```python
from build123d import *

# Parameters (mm, degrees)
F0_R     = 8
F1_DEPTH = 49
F3_D     = 4.2
F3_DEPTH = 17.4
F3_TIP   = 1.2618073
F5_D     = 4.2
F5_DEPTH = 17.4
F5_TIP   = 1.2618073


with BuildPart() as f1:
    # F0 (on Top) → F1 (new body)
    with BuildSketch(Plane.XY):
        Circle(F0_R)
    extrude(amount=F1_DEPTH)

    # F3
    with Locations(Plane.XY.offset(49)):
        with Locations((0, 0)):
            Hole(F3_D / 2, depth=F3_DEPTH)
            with Locations((0, 0, -(F3_DEPTH + F3_TIP / 2))):  # 118° drill point
                Cone(0, F3_D / 2, F3_TIP, mode=Mode.SUBTRACT)

    # F5
    with Locations(Plane(origin=(0, 0, 0), x_dir=(1, 0, 0), z_dir=(0, 0, -1))):
        with Locations((0, 0)):
            Hole(F5_D / 2, depth=F5_DEPTH)
            with Locations((0, 0, -(F5_DEPTH + F5_TIP / 2))):  # 118° drill point
                Cone(0, F5_D / 2, F5_TIP, mode=Mode.SUBTRACT)


solid = f1.part
```
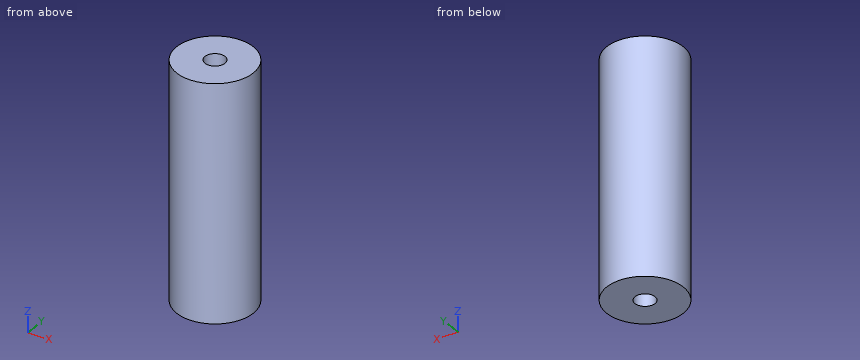
Geometry: final body of the model. Coordinates: model frame, mm. Coordinates: 2 decimals unless noted, no trailing zeros. Order: outer loops, then holes, each group sorted by start corner. A loop starts at its lowest first (then second) coordinate and runs counter-clockwise, first axis right, second up.
Item 1: Section query B-B (y = 5.25). Output: boundary loops of the cut face in (x, z), then the cut area to 3 significant figures.
Answer:
outline: (-6.04, 0) - (6.04, 0) - (6.04, 49) - (-6.04, 49) - close
area: 592 mm2
Item 2: Section query A-A (x = 6.5). Output: boundary loops of the cut face in (y, z), then the cut area to 3 significant figures.
Answer:
outline: (-4.66, 0) - (4.66, 0) - (4.66, 49) - (-4.66, 49) - close
area: 457 mm2
Item 3: Contact query for flat-ended pins moving along their axis: P1, Ø2.5, axis at x = 0, y = 0, coming from the -Z side; P2, Ø2, axis at x = -5, z = 10.5, coming from the -Y side; P3, Ø1, axis at x = -2.5, z = 35.5, coming from the -Y side. Output: stop coordinate, or through.
Answer:
P1: stops at z = 17.91
P2: stops at y = -6.93
P3: stops at y = -7.75
Item 4: Material intervals for line 1 along Y through (x, z) = (0, 43); line 2 along Y through (x, z) = (0.75, 6); line 3 along X through (y, z) = (-5.5, 7), sorted ascending.
Answer:
line 1: y = -8 to -2.1, 2.1 to 8
line 2: y = -7.96 to -1.96, 1.96 to 7.96
line 3: x = -5.81 to 5.81
